```python
from build123d import *

# Parameters (mm, degrees)
SKETCH_R        = 16
SKETCH_R_2      = 2.25
PAD_DEPTH       = 6.3
SKETCH003_R     = 3.1
POCKET_DEPTH    = 6
SKETCH004_R     = 6.5
POCKET001_DEPTH = 2
SKETCH005_R     = 0.85
POCKET002_DEPTH = 6


with BuildPart() as part:
    # Sketch → Pad (new body)
    with BuildSketch(Plane.XY):
        Circle(SKETCH_R)
        with Locations((-3.25, 0)):
            Circle(SKETCH_R_2, mode=Mode.SUBTRACT)
        with Locations((3.25, 0)):
            Circle(SKETCH_R_2, mode=Mode.SUBTRACT)
    extrude(amount=PAD_DEPTH)

    # Sketch003 (on Face5 of Pad) → Pocket (cut)
    with BuildSketch(Plane.XY.offset(6.3)):
        with Locations((9.526279, 5.5)):
            Circle(SKETCH003_R)
        with Locations((3.762222, 10.336619)):
            Circle(SKETCH003_R)
        with Locations((-3.762222, 10.336619)):
            Circle(SKETCH003_R)
        with Locations((-9.526279, 5.5)):
            Circle(SKETCH003_R)
        with Locations((-10.832885, -1.91013)):
            Circle(SKETCH003_R)
        with Locations((-7.070664, -8.426489)):
            Circle(SKETCH003_R)
        with Locations((0, -11)):
            Circle(SKETCH003_R)
        with Locations((7.070664, -8.426489)):
            Circle(SKETCH003_R)
        with Locations((10.832885, -1.91013)):
            Circle(SKETCH003_R)
    extrude(amount=-POCKET_DEPTH, mode=Mode.SUBTRACT)

    # Sketch004 (on Face3 of Pocket) → Pocket001 (cut)
    with BuildSketch(Plane.XY.offset(6.3)):
        Circle(SKETCH004_R)
    extrude(amount=-POCKET001_DEPTH, mode=Mode.SUBTRACT)

    # Sketch005 (on Face3 of Pocket001) → Pocket002 (cut)
    with BuildSketch(Plane.XY.offset(6.3)):
        with Locations((3.32265, -4)):
            Circle(SKETCH005_R)
        with Locations((-3.32265, 4)):
            Circle(SKETCH005_R)
    extrude(amount=-POCKET002_DEPTH, mode=Mode.SUBTRACT)


solid = part.part
```
Check sheet for the modelled part. Datum: model origin and axes. Units: mm. A direction names the side the tool comes from. Give positions to 0.01 mm unless a question says otherwise; leave off trailing zeros. Order: outer loops, then holes, each group sorted by start corner. A loop starts at its lowest first (then second) coordinate and runs counter-clockwise, first axis right, second up. Notation, with made-up numbers: (13, 72) -> (27, 72) arc R34 ccw to (27, 108) -> close; hole circle Ø4 at (74.5, 85.25). An arc over 180 degrees is marked (long way). Use CSV: the item, a comma, the result in double quotes. Start each with the question number.
1) Sectioned sample at A-A, the plane y = 0. Record the boundary of the cut face in (x, z).
2) Go/stop test with flat-tipped pins: P1, Ø1.4, axis at x = 3.32, y = -4, coming from the +Z side; P2, Ø1, axis at y = 9.5, z = 5.5, coming from the +X side; P3, Ø2, axis at y = 11, z = 4.5, coming from the +X side. Record where each tip stops, or that it passes through.
3) Mould release check, pull along Y, two halves, no side actions. Record for faces 1 (the face through (13.79, -0.98, 3.34)), 2 (the face through (0, 0, 0)), 3 (the face through (7, -8, 0.3)): released by +Y, released by -Y, zero draft, split by the parting line, or undercut.
4) Material ranges on line 1 (Y direction, x = -9, z = 3.25) (3 decimals); line 2 (Y direction, x = -3.5, z = 2); line 3 (X direction, y = -3, z = 5), recorded low to high. Write a range as from..to.
5) Sectioned sample at B-B, the plane z = 5.75. Give the number of separate pieces and of enclosed holes in the cut face, plus the area to 3 significant figures.
6) Set-up check for faces 4 (the face through (-7, -8, 0.3)), 5 (the face through (2.96, 2.23, 2.12)): record each of +Z, -Z, +X, -X, +Y, -Y from which the full face is reachable in a straight line by a thin tool's end or side.
7) Sectioned sample at D-D, the plane y = 8. Record the boundary of the cut face in (x, z).
8) Sectioned sample at C-C, the plane x = 0. Record the boundary of the cut face in (y, z), plus the area to 3 significant figures.
Recorded:
1,outline,"(-16, 0) -> (-5.5, 0) -> (-5.5, 4.3) -> (-6.5, 4.3) -> (-6.5, 6.3) -> (-8.39, 6.3) -> (-8.39, 0.3) -> (-13.27, 0.3) -> (-13.27, 6.3) -> (-16, 6.3) -> close; (-1, 0) -> (1, 0) -> (1, 4.3) -> (-1, 4.3) -> close; (5.5, 0) -> (16, 0) -> (16, 6.3) -> (13.27, 6.3) -> (13.27, 0.3) -> (8.39, 0.3) -> (8.39, 6.3) -> (6.5, 6.3) -> (6.5, 4.3) -> (5.5, 4.3) -> close"
2,P1,"z = 0.3"
2,P2,"x = 13.23"
2,P3,"x = 12.49"
3,face 1,"undercut"
3,face 2,"zero draft"
3,face 3,"undercut"
4,line 1,"-13.229..-10.853, -6..-4.41, 0.59..2.445, 8.555..13.229"
4,line 2,"-15.61..-2.24, 2.24..3.17, 4.83..7.25, 13.43..15.61"
4,line 3,"-15.72..-13.73, -7.93..-5.77, 5.77..7.93, 13.73..15.72"
5,separate pieces,"1"
5,enclosed holes,"10"
5,area,"400 mm2"
6,face 4,"+Z"
6,face 5,"+Z, -Z"
7,outline,"(-13.86, 0) -> (13.86, 0) -> (13.86, 6.3) -> (11.36, 6.3) -> (11.36, 0.3) -> (7.69, 0.3) -> (7.69, 6.3) -> (5.8, 6.3) -> (5.8, 0.3) -> (1.73, 0.3) -> (1.73, 6.3) -> (-1.73, 6.3) -> (-1.73, 0.3) -> (-5.8, 0.3) -> (-5.8, 6.3) -> (-7.69, 6.3) -> (-7.69, 0.3) -> (-11.36, 0.3) -> (-11.36, 6.3) -> (-13.86, 6.3) -> close"
8,outline,"(-16, 0) -> (16, 0) -> (16, 6.3) -> (6.5, 6.3) -> (6.5, 4.3) -> (-6.5, 4.3) -> (-6.5, 6.3) -> (-7.9, 6.3) -> (-7.9, 0.3) -> (-14.1, 0.3) -> (-14.1, 6.3) -> (-16, 6.3) -> close"
8,area,"138 mm2"
